```python
from build123d import *

# Parameters (mm, degrees)
POGO_R              = 0.75
POGO_W              = 19.9
POGO_H              = 24.9
BOSS_EXTRUDE1_DEPTH = 5.5


with BuildPart() as part:
    # pogo → Boss-Extrude1 (new body)
    with BuildSketch(Plane.XY):
        with BuildLine():
            Line((-12.95, 15.45), (0.55, 15.45))
            Line((0.55, 15.45), (0.55, 14.15))
            ThreePointArc((0.55, 14.15), (1.35, 13.45), (2.05, 14.25))
            Line((2.05, 14.25), (2.05, 15.45))
            Line((2.05, 15.45), (12.95, 15.45))
            Line((12.95, 15.45), (12.95, -15.45))
            Line((12.95, -15.45), (-12.95, -15.45))
            Line((-12.95, -15.45), (-12.95, 15.45))
        make_face()
        with Locations((-11.5, 13)):
            Circle(POGO_R, mode=Mode.SUBTRACT)
        with Locations((11.5, 13)):
            Circle(POGO_R, mode=Mode.SUBTRACT)
        with Locations((11.5, 11)):
            Circle(POGO_R, mode=Mode.SUBTRACT)
        with Locations((11.5, 9)):
            Circle(POGO_R, mode=Mode.SUBTRACT)
        with Locations((11.5, 7)):
            Circle(POGO_R, mode=Mode.SUBTRACT)
        with Locations((11.5, 5)):
            Circle(POGO_R, mode=Mode.SUBTRACT)
        with Locations((11.5, 3)):
            Circle(POGO_R, mode=Mode.SUBTRACT)
        with Locations((11.5, 1)):
            Circle(POGO_R, mode=Mode.SUBTRACT)
        with Locations((11.5, -1)):
            Circle(POGO_R, mode=Mode.SUBTRACT)
        with Locations((11.5, -3)):
            Circle(POGO_R, mode=Mode.SUBTRACT)
        with Locations((11.5, -5)):
            Circle(POGO_R, mode=Mode.SUBTRACT)
        with Locations((11.5, -7)):
            Circle(POGO_R, mode=Mode.SUBTRACT)
        with Locations((11.5, -9)):
            Circle(POGO_R, mode=Mode.SUBTRACT)
        with Locations((11.5, -11)):
            Circle(POGO_R, mode=Mode.SUBTRACT)
        with Locations((11.5, -13)):
            Circle(POGO_R, mode=Mode.SUBTRACT)
        with Locations((-11.5, 11)):
            Circle(POGO_R, mode=Mode.SUBTRACT)
        with Locations((-11.5, 9)):
            Circle(POGO_R, mode=Mode.SUBTRACT)
        with Locations((-11.5, 7)):
            Circle(POGO_R, mode=Mode.SUBTRACT)
        with Locations((-11.5, 5)):
            Circle(POGO_R, mode=Mode.SUBTRACT)
        with Locations((-11.5, 3)):
            Circle(POGO_R, mode=Mode.SUBTRACT)
        with Locations((-11.5, 1)):
            Circle(POGO_R, mode=Mode.SUBTRACT)
        with Locations((-11.5, -1)):
            Circle(POGO_R, mode=Mode.SUBTRACT)
        with Locations((-11.5, -3)):
            Circle(POGO_R, mode=Mode.SUBTRACT)
        with Locations((-11.5, -5)):
            Circle(POGO_R, mode=Mode.SUBTRACT)
        with Locations((-11.5, -7)):
            Circle(POGO_R, mode=Mode.SUBTRACT)
        with Locations((-11.5, -9)):
            Circle(POGO_R, mode=Mode.SUBTRACT)
        with Locations((-11.5, -11)):
            Circle(POGO_R, mode=Mode.SUBTRACT)
        with Locations((-11.5, -13)):
            Circle(POGO_R, mode=Mode.SUBTRACT)
        with Locations((-9, 14)):
            Circle(POGO_R, mode=Mode.SUBTRACT)
        with Locations((-7, 14)):
            Circle(POGO_R, mode=Mode.SUBTRACT)
        with Locations((-5, 14)):
            Circle(POGO_R, mode=Mode.SUBTRACT)
        with Locations((-3, 14)):
            Circle(POGO_R, mode=Mode.SUBTRACT)
        with Locations((-1, 14)):
            Circle(POGO_R, mode=Mode.SUBTRACT)
        with Locations((3, 14)):
            Circle(POGO_R, mode=Mode.SUBTRACT)
        with Locations((5, 14)):
            Circle(POGO_R, mode=Mode.SUBTRACT)
        with Locations((7, 14)):
            Circle(POGO_R, mode=Mode.SUBTRACT)
        with Locations((9, 14)):
            Circle(POGO_R, mode=Mode.SUBTRACT)
        with Locations((-7, -14)):
            Circle(POGO_R, mode=Mode.SUBTRACT)
        with Locations((-5, -14)):
            Circle(POGO_R, mode=Mode.SUBTRACT)
        with Locations((3, -14)):
            Circle(POGO_R, mode=Mode.SUBTRACT)
        with Locations((5, -14)):
            Circle(POGO_R, mode=Mode.SUBTRACT)
        with Locations((7, -14)):
            Circle(POGO_R, mode=Mode.SUBTRACT)
        with Locations((9, -14)):
            Circle(POGO_R, mode=Mode.SUBTRACT)
        with Locations((-9, -14)):
            Circle(POGO_R, mode=Mode.SUBTRACT)
        Rectangle(POGO_W, POGO_H, mode=Mode.SUBTRACT)
    extrude(amount=BOSS_EXTRUDE1_DEPTH)


solid = part.part
```
CAD build for the part. Positions are in the model's coordinates, mm. A direction names the side the tool comes from. Coordinates: 2 decimals unless noted, no trailing zeros. Order: outer loops, then holes, each group sorted by start corner. A loop starts at its lowest first (then second) coordinate and runs counter-clockwise, first axis right, second up. Notation, with made-up numbers: (-16, 12) - (-7, 12) arc R26 ccw to (-7, 49) - close; hole circle Ø4 at (28, 12.25). An arc over 180 degrees is marked (long way). Answer in a Markdown table with one row per item.
1. Flat gauge pins, fed straight in: P1, Ø1.7, axis at x = 11.5, y = -9, coming from the +Z side; P2, Ø1.4, axis at x = 11.5, y = 13, coming from the +Z side. Where does each tip first touch, or does it go through?
Answer:
| item | result |
|---|---|
| P1 | z = 5.5 |
| P2 | through |
2. Slice it at B-B, the plane y = 9. List the corners of the cut face in (x, z).
Answer:
| item | result |
|---|---|
| outline | (-12.95, 0) - (-12.25, 0) - (-12.25, 5.5) - (-12.95, 5.5) - close; (-10.75, 0) - (-9.95, 0) - (-9.95, 5.5) - (-10.75, 5.5) - close; (9.95, 0) - (10.75, 0) - (10.75, 5.5) - (9.95, 5.5) - close; (12.25, 0) - (12.95, 0) - (12.95, 5.5) - (12.25, 5.5) - close |
3. 3-axis set-ups, long thin cutter, end or side, ignore diameter. For faces 1 (the face through (0, -12.45, 3)), 2 (the face through (-6, 15.45, 3)): which of +Z, -Z, +X, -X, +Y, -Y reach the whole face in a straight line?
Answer:
| item | result |
|---|---|
| face 1 | +Z, -Z |
| face 2 | +Z, -Z, +X, -X, +Y |
4. Slice it at D-D, the plane z = 4.1. Give the number of separate pieces and of enclosed holes in the cut face, then the cut area to 3 significant figures.
Answer:
| item | result |
|---|---|
| separate pieces | 1 |
| enclosed holes | 45 |
| area | 224 mm² |
5. Slice it at C-C, the plane x = -1. List the corners of the cut face in (y, z).
Answer:
| item | result |
|---|---|
| outline | (-15.45, 0) - (-12.45, 0) - (-12.45, 5.5) - (-15.45, 5.5) - close; (12.45, 0) - (13.25, 0) - (13.25, 5.5) - (12.45, 5.5) - close; (14.75, 0) - (15.45, 0) - (15.45, 5.5) - (14.75, 5.5) - close |
6. Slice it at A-A, the plane x = 7. List the corners of the cut face in (y, z), then the cut area to 3 significant figures.
Answer:
| item | result |
|---|---|
| outline | (-15.45, 0) - (-14.75, 0) - (-14.75, 5.5) - (-15.45, 5.5) - close; (-13.25, 0) - (-12.45, 0) - (-12.45, 5.5) - (-13.25, 5.5) - close; (12.45, 0) - (13.25, 0) - (13.25, 5.5) - (12.45, 5.5) - close; (14.75, 0) - (15.45, 0) - (15.45, 5.5) - (14.75, 5.5) - close |
| area | 16.5 mm² |
7. Drill centre lines: L1, parallel to Y at x = 7, z = 3.8; L2, parallel to Y at x = 6, z = 0.5; L3, parallel to X at y = 11.5, z = 3.1. Where is each one in solid material? Low to high. Write a range as from..to.
Answer:
| item | result |
|---|---|
| L1 | -15.45..-14.75, -13.25..-12.45, 12.45..13.25, 14.75..15.45 |
| L2 | -15.45..-12.45, 12.45..15.45 |
| L3 | -12.95..-12.06, -10.94..-9.95, 9.95..10.94, 12.06..12.95 |
8. Pull direction X, two halves, no side cores. Call faces 3 (the face through (10.905, -5.456, 2.712)), 4 (the face through (12.95, 0, 3)), 5 (the face through (-12.95, 0, 3)): +X half, -X half, draft (parallel to the pull), parting line (faces both ways), or undercut.
Answer:
| item | result |
|---|---|
| face 3 | undercut |
| face 4 | +X half |
| face 5 | -X half |
